Autodesk Inventor part; units mm, degrees
ref_plane "YZ Plane" through (0, 0, 0) normal (1, 0, 0) x (0, 1, 0)
ref_plane "XZ Plane" through (0, 0, 0) normal (0, 1, 0) x (-1, 0, 0)
ref_plane "XY Plane" through (0, 0, 0) normal (0, 0, 1) x (1, 0, 0)
sketch "Sketch1" plane through (0, 0, 0) normal (0, 1, 0) x (-1, 0, 0)
  arc A0 (3.9007, 1.0556) -> (2.1982, -3.3894) centre (0.0024, 0.0001) ccw
  arc A1 (19.0232, 1.0556) -> (-16.4856, -9.5418) centre (0.0024, 0.0001) ccw
  line L0 (3.9007, 1.0556) -> (19.0232, 1.0556)
  line L1 (2.1982, -3.3894) -> (19.0232, -3.3894)
  line L2 (19.0232, -7.0431) -> (11.658, -7.0431)
  line L3 (19.0232, -3.3894) -> (19.0232, -7.0431)
  arc A2 (-16.4856, -9.5418) -> (7.4534, -10.991) centre (-3.9181, -0.3889) ccw
  line L4 (19.0232, 1.0556) -> (19.0232, 51.8556)
  line L5 (-19.0476, 0.0001) -> (-19.0476, 51.8556)
  line L6 (-19.0476, 0.0001) -> (-19.4605, 0.0001)
  arc A3 (19.0232, 51.8556) -> (-64.3153, 200.5038) centre (-187.3249, 33.8538) ccw
  arc A4 (-19.0476, 51.5998) -> (-53.7472, 153.729) centre (-221.3606, 39.8209) ccw
  line L7 (9.8792, 51.4484) -> (9.8792, 35.8565)
  arc A5 (-10.1576, 51.8556) -> (-53.8573, 169.027) centre (-221.3606, 39.8209) ccw
  line L8 (-10.1576, 51.8556) -> (-10.1576, 35.8565)
  line L9 (9.8792, 23.8284) -> (-10.1576, 23.8284) construction
  line L10 (9.8792, 23.8284) -> (29.9159, 23.8284) construction
  arc A6 (4.8483, 29.6451) -> (9.8792, 35.8565) centre (3.5292, 35.8565) ccw
  arc A7 (-10.1576, 35.8565) -> (-5.1267, 29.6451) centre (-3.8076, 35.8565) ccw
  line L11 (4.8483, 29.6451) -> (-5.1267, 29.6451)
  arc A8 (19.0232, 51.8556) -> (-64.3153, 200.5038) centre (-187.3249, 33.8538) ccw
  arc A9 (-31.6355, 156.1642) -> (-40.7288, 149.9287) centre (-26.0329, 138.2456) ccw
  arc A10 (-25.3873, 119.4827) -> (-11.9806, 125.796) centre (-26.0329, 138.2456) ccw
  arc A11 (-7.259, 116.1658) -> (-22.0111, 110.6115) centre (-7.259, 93.7981) ccw
  arc A12 (-12.2768, 72.0005) -> (6.1478, 75.8935) centre (-7.259, 93.7981) ccw
  arc A13 (8.4637, 63.2789) -> (-11.0177, 62.3465) centre (-0.1392, 39.0411) ccw
  arc A14 (-44.388, 155.7184) -> (-36.6502, 162.2912) centre (-47.9514, 167.7544) ccw
  line L12 (7.4534, -9.5831) -> (7.4534, -10.991)
  line L13 (11.658, -7.0431) -> (9.9934, -7.0431)
  line L14 (9.9934, -7.0431) -> (7.4534, -7.0431)
  line L15 (7.4534, -7.0431) -> (7.4534, -9.5831)
  line L16 (-53.7472, 153.729) -> (-70.9133, 191.6752)
  arc A15 (-64.3153, 200.5038) -> (-70.9133, 191.6752) centre (-63.9188, 193.3277) ccw
  arc A16 (-53.8573, 169.027) -> (-46.1861, 172.7021) centre (-51.6725, 174.3104) ccw
  arc A17 (9.8792, 51.4484) -> (-46.1861, 172.7021) centre (-187.3249, 33.8538) ccw
  point P0 (-0.1392, 29.6451)
  point P1 (19.0232, 1.0556)
  point P2 (-64.3153, 200.5038)
  point P3 (7.4534, 1.0556)
  dimension "d17" = 8.0772
  dimension "d19" = 4.445
  dimension "d22" = 50.8
  dimension "d27" = 8.89
  dimension "d28" = 8.89
  dimension "d31" = 180
  dimension "d32" = 6.35
  dimension "d33" = 207.1318
  dimension "d34" = 33.8537
  dimension "d35" = 29.6449
  dimension "d36" = 19.05
  dimension "d37" = 3.3895
extrude "Extrusion1" add sketch "Sketch1" along normal blind 19.05 contours A0 L1 L3 L2 L13 L14 L15 L12 A2 A1 L0 | A1 L5 A4 L16 A15 A3 L4 | A13 A5 A12 A17 | A11 A5 A10 A17 | A9 A5 A14 A17
fillet "Fillet1" radius 1.27 1 edges at (-7.4534, 9.525, -7.0431)
sketch "Sketch2" plane through (-19.0232, 0, -7.0431) normal (0, 0, -1) x (-1, 0, 0)
  line L0 (0, 0) -> (0, 19.05)
  line L1 (-10.2998, 19.05) -> (0, 19.05)
  point P0 (-19.0232, 0)
  point P1 (-5.08, 9.525)
  point P2 (0, 9.525)
  point P3 (-5.1499, 19.05)
  dimension "d44" = 5.08
  dimension "d45" = 9.525
hole "Hole1" at (-13.9432, 9.525, -7.0431) direction (0, 0, 1) diameter 5.334 end up to surface
sketch "Sketch3" plane through (-3.9007, 0, 1.0556) normal (0, 0, -1) x (-1, 0, 0)
  circle A0 centre (10.0425, 9.525) radius 2.667
  point P0 (-3.9007, 0)
hole "Hole2" at (-13.9432, 9.525, 1.0556) direction (0, 0, 1) diameter 5.588 depth 10.16
sketch "Sketch4" plane through (-19.0232, 0, 1.0556) normal (-1, 0, 0) x (0, 0, 1)
  line L0 (0, 6.731) -> (0, 12.319)
  line L1 (10.16, 12.319) -> (10.16, 6.731)
  line L2 (0, 6.731) -> (5.08, 6.731)
  line L3 (10.16, 6.731) -> (0, 6.731)
  line L4 (0, 12.319) -> (5.08, 12.319)
  line L5 (10.16, 12.319) -> (0, 12.319)
  line L6 (0, 0) -> (50.8, 0)
  line L7 (0, 9.525) -> (16.1442, 9.525) construction
  line L8 (5.08, 9.525) -> (5.08, 2.921)
  line L9 (5.08, 9.525) -> (5.08, 16.129)
  line L10 (5.08, 16.129) -> (22.86, 16.129)
  line L11 (22.86, 16.129) -> (22.86, 2.921)
  line L12 (22.86, 2.921) -> (5.08, 2.921)
  point P0 (-1.0556, 0)
  dimension "d63" = 5.08
  dimension "d65" = 6.604
  dimension "d66" = 6.604
  dimension "d67" = 17.78
extrude "Extrusion2" cut sketch "Sketch4" against normal blind 11.43 contours L8 L9 L5 L1 L3 | L3 L1 L5 L9 L10 L11 L12 L8
sketch "Sketch6" plane through (0, 0, 0) normal (0, -1, 0) x (1, 0, 0)
  circle A0 centre (-0.4283, -8.8611) radius 1.27
  circle A1 centre (9.6886, 9.5689) radius 3.81
  arc A2 (-0.3421, -7.594) -> (6.8398, 7.039) centre (0.2554, 1.1917) ccw
  arc A3 (-0.7205, -10.097) -> (12.5379, 12.0984) centre (2.3988, 3.0973) ccw
  arc A4 (-7.4534, -10.991) -> (16.4856, -9.5418) centre (3.9181, -0.3889) ccw
  line L0 (-9.198, -6.9778) -> (-6.15, -6.9778)
  line L1 (-6.15, -6.9778) -> (-6.15, -12.2358)
  line L2 (-6.15, -12.2358) -> (-9.198, -12.2358)
  line L3 (-9.198, -12.2358) -> (-9.198, -6.9778)
  point P0 (0, 0)
  dimension "d90" = 3.048
  dimension "d91" = 2.54
extrude "Extrusion4" cut sketch "Sketch6" against normal blind 25.4
fillet "Fillet2" radius 3.175 1 edges at (-6.15, 9.525, -6.9778)
fillet "Fillet3" radius 3.175 1 edges at (-6.15, 9.525, -12.2358)
sketch "Sketch9" plane through (0, 0, 0) normal (0, -1, 0) x (1, 0, 0)
  point P0 (0, 0)
sketch "Sketch7" plane through (0, 0, 0) normal (0, -1, 0) x (1, 0, 0)
  circle A0 centre (0, 0) radius 5.1181
  dimension "d96" = 10.2362
sketch "Sketch8" plane through (0, 0, 0) normal (0, -1, 0) x (1, 0, 0)
  arc A0 (-3.835, -3.3894) -> (-5.0081, 1.0556) centre (0, 0) ccw
  arc A1 (-0.3421, -7.594) -> (6.8398, 7.039) centre (0.2554, 1.1917) ccw
  arc A2 (12.5379, 12.0984) -> (6.8398, 7.039) centre (9.6886, 9.5689) ccw
  arc A3 (-0.7205, -10.097) -> (12.5379, 12.0984) centre (2.3988, 3.0973) ccw
  arc A4 (-0.3421, -7.594) -> (-0.7205, -10.097) centre (-0.4283, -8.8611) ccw
  circle A5 centre (9.6886, 9.5689) radius 3.81
  circle A6 centre (-0.4283, -8.8611) radius 1.27
  arc A7 (-0.3421, -7.594) -> (6.8398, 7.039) centre (1.573, 0.545) ccw
  point P0 (0.0088, -7.6687)
  point P1 (7.474, 6.4687)
  point P2 (6.8398, 7.039)
  point P3 (-0.3421, -7.594)
properties part number "Central Claw V2_3DPrint"
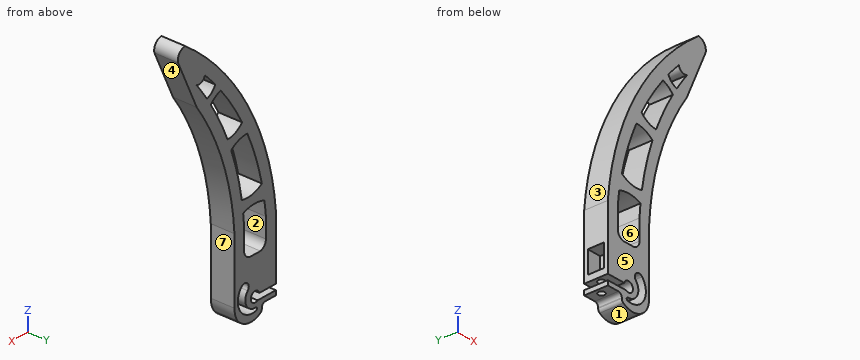
Input: part model. Units: mm. Frame: model coordinates. Face numbers are marked on the shaded views. A direction names the side the tool comes from. Give positions to 0.01 mm unless a question says otherwise; leave off trailing zeros. Order: outer loops, then holes, each group sorted by start corner. A loop starts at its lowest first (then second) coordinate and runs counter-clockwise, first axis right, second up. Notation, with made-up numbers: M 20.25,8 L 71.25,8 A26 cw 71.25,46 Z; hole C 16.25,61.25 d2. An arc over 180 degrees is marked long. One line per question, with ' | ' between items. Start each with the question number.
1. Section query A-A (z = 45). Return the cut outline in (x, y).
2. Section query C-C (y = 9.25). Count the separate pieces of the cut face and the enclosed holes in it, and give its area (3 significant figures).
3. First-contact query: pin 1 Ø4 at (y, z) = (4, 76.5) entering from +X; pin 2 Ø8 at (x, z) = (6.5, 60.5) entering from +Y; pin 3 Ø11 at (x, y) = (-14.5, 7) entering from -Z; pin 4 Ø8 at (x, y) = (47, 11.5) entering from -Z. Flat tips, straight axial feed; report the tip coordinate or a pass-through.
4. Material intervals for probe 1 along X at (y, z) = (7.75, -6); probe 2 along Z at (x, y) = (39.5, 3); probe 3 along Z at (x, y) = (48, 11.5), sorted ascending. Write a range as [from, to].
5. Pull-direction query (X, two-part tool) for the marked faces 1, 2, 3 and 4; classes: released by +X, released by -X, zero draft, split by the parting line, or undercut.
6. Access query for the marked faces 5, 6 and 7. Directions: +Z, -Z, +X, -X, +Y, -Y. A direction counts if a zero-diameter tool reaches every point of the face in a straight line with its end or side. Return the directions, or none.
7. Section query B-B (x = 49). Return the cut outline in (y, z), and give its area (3 significant figures).
Here are the results:
1) outline: M -19.02,0 L -9.88,0 L -9.88,19.05 L -19.02,19.05 Z; M 10.16,0 L 19.05,0 L 19.05,19.05 L 10.16,19.05 Z
2) separate pieces: 3 | enclosed holes: 5 | area: 4,720 mm²
3) pin 1: x = 22.43 | pin 2: y = 19.05 | pin 3: z = -7.04 | pin 4: z = 136.03
4) probe 1: [-19.02, -15.93], [-11.95, 5.34], [12.45, 18.08] | probe 2: [129.24, 147.89], [151.33, 158.47], [165.56, 178.94] | probe 3: [144.78, 161.05], [169.93, 187.13]
5) face 1: split by the parting line | face 2: undercut | face 3: released by -X | face 4: released by +X
6) face 5: +Z, -Z, +X, -X, -Y | face 6: +Y, -Y | face 7: -Z, +X, +Y, -Y
7) outline: M 0,146.41 L 19.05,146.41 L 19.05,162.47 L 0,162.47 Z; M 0,169.26 L 19.05,169.26 L 19.05,188.03 L 0,188.03 Z | area: 664 mm²
